Read the model definition and answer for the solid it produces. Units are mm, in the model's axes. A direction names the side the tool comes from. Give positions to 0.01 mm unless a question says otherwise; leave off trailing zeros. Write each loop counter-clockwise with the first axis right and the second up, starting at its lowest first coordinate (ties: lowest second). Pieces come first, ordered by that corner, then holes. Notation, with made-up numbers: (60.5, 29.5) - (90.5, 29.5) arc R21 ccw to (90.5, 45.5) - close; hole circle Ø11 at (-14, 60). An arc over 180 degrees is marked (long way). Answer as a JSON object with one key per item and string values. Group by question number.
Autodesk Inventor part; units mm, degrees
ref_plane "YZ Plane" through (0, 0, 0) normal (1, 0, 0) x (0, 1, 0)
ref_plane "XZ Plane" through (0, 0, 0) normal (0, 1, 0) x (-1, 0, 0)
ref_plane "XY Plane" through (0, 0, 0) normal (0, 0, 1) x (1, 0, 0)
sketch "Sketch2" plane through (0, 0, 0) normal (0, 0, 1) x (1, 0, 0)
  circle A0 centre (0, 0) radius 10
  dimension "d7" = 20
extrude "Extrusion2" add sketch "Sketch2" along normal blind 25
sketch "Sketch3" plane through (0, 0, 25) normal (0, 0, 1) x (1, 0, 0)
  circle A0 centre (0, 0) radius 4.1
  dimension "d10" = 8.2
extrude "Extrusion3" cut sketch "Sketch3" against normal blind 10
thread "Thread1"
sketch "Sketch4" plane through (0, 0, 0) normal (0, 0, -1) x (-1, 0, 0)
  circle A0 centre (0, 0) radius 2.6
  dimension "d15" = 5.2
extrude "Extrusion4" cut sketch "Sketch4" against normal blind 15.175
thread "Thread2"
chamfer "Chamfer1" distance 0.2 angle 45 1 edges at (-10, 0, 25)
chamfer "Chamfer2" distance 0.2 angle 45 1 edges at (-10, 0, 0)
sketch "Sketch5" plane through (0, 0, 0) normal (0, 1, 0) x (-1, 0, 0)
  point P0 (0, 0)
  point P1 (10, 0.2)
sketch "Sketch6" plane through (0, 0, 25) normal (0, 0, 1) x (1, 0, 0)
  circle A0 centre (0, 0) radius 4.5065
extrude "Extrusion5" cut sketch "Sketch6" against normal blind 0.2
sketch "Sketch7" plane through (0, 0, 0) normal (0, 0, -1) x (-1, 0, 0)
  circle A0 centre (0, 0) radius 3.1378
extrude "Extrusion6" cut sketch "Sketch7" against normal blind 0.2
sketch "Sketch8" plane through (0, 0, 25) normal (0, 0, 1) x (1, 0, 0)
  point P0 (0, 0)
sketch "Sketch9" plane through (0, 0, 25) normal (0, 0, 1) x (1, 0, 0)
  point P0 (0, 0)
sketch "Sketch10" plane through (0, 0, 25) normal (0, 0, 1) x (1, 0, 0)
  point P0 (0, 0)
properties part number "coupler"
1) Find section D-D, the plane z = 23.75. Write down the section's boundary in (x, y), and give its area (3 significant figures).
2) Flat-ended cylindrical pins translate along their axes: pin 1 Ø2.5 at (x, y) = (-0.5, -2) entering from +Z; pin 2 Ø1 at (x, z) = (1.5, 4) entering from -Y; pin 3 Ø1 at (x, z) = (-3.5, 13) entering from -Y; pin 4 Ø4 at (x, y) = (0, 0) entering from +Z. Find the tip coordinate at first contact, or state that the pin passes through.
3) Find section A-A, the plane x = 0. Write down the section's boundary in (y, z), and give its area (3 significant figures).
4) Find section C-C, the plane z = 7.5. Write down the section's boundary in (x, y), and give its area (3 significant figures).
5) Find the intervals of material crossed by line 1 (Y direction, x = 0, z = 5.5); line 2 (Y direction, x = 0, z = 22.25); line 3 (Z direction, x = -0.5, y = 3.25), in increasing order. Write a range as [from, to].
6) Which of the six approach directions +Z, -Z, +X, -X, +Y, -Y give full straight-line access (tool end or side, diameter ignored) to faces 1 (the cylindrical face through (-0.534, 4.065, 19.969)), 2 (the cylindrical face through (0.338, 2.578, 7.496))?
7) For a pull along X with two mould halves and no side action, classify faces 3 (the flat face through (2, 2, 0.2)), 4 (the cylindrical face through (-2.17, 9.76, 12.33)), 5 (the flat face through (4, 0, 0)) as released by +X, released by -X, zero draft, split by the parting line, or undercut.
Values follow:
{
 "1": {"outline": "circle Ø20 at (0, 0); hole circle Ø8.2 at (0, 0)", "area": "261 mm2"},
 "2": {"pin 1": "stops at z = 15", "pin 2": "stops at y = -9.95", "pin 3": "stops at y = -9.54", "pin 4": "passes through"},
 "3": {"outline": "(-10, 0.2) - (-9.8, 0) - (-3.14, 0) - (-3.14, 0.2) - (-2.6, 0.2) - (-2.6, 15) - (-4.1, 15) - (-4.1, 24.8) - (-4.51, 24.8) - (-4.51, 25) - (-9.8, 25) - (-10, 24.8) - close; (2.6, 0.2) - (3.14, 0.2) - (3.14, 0) - (9.8, 0) - (10, 0.2) - (10, 24.8) - (9.8, 25) - (4.51, 25) - (4.51, 24.8) - (4.1, 24.8) - (4.1, 15) - (2.6, 15) - close", "area": "340 mm2"},
 "4": {"outline": "circle Ø20 at (0, 0); hole circle Ø5.2 at (0, 0)", "area": "293 mm2"},
 "5": {"line 1": "y = [-10, -2.6], [2.6, 10]", "line 2": "y = [-10, -4.1], [4.1, 10]", "line 3": "z = [0, 15]"},
 "6": {"face 1": "+Z", "face 2": "+Z, -Z"},
 "7": {"face 3": "undercut", "face 4": "split by the parting line", "face 5": "zero draft"}
}
